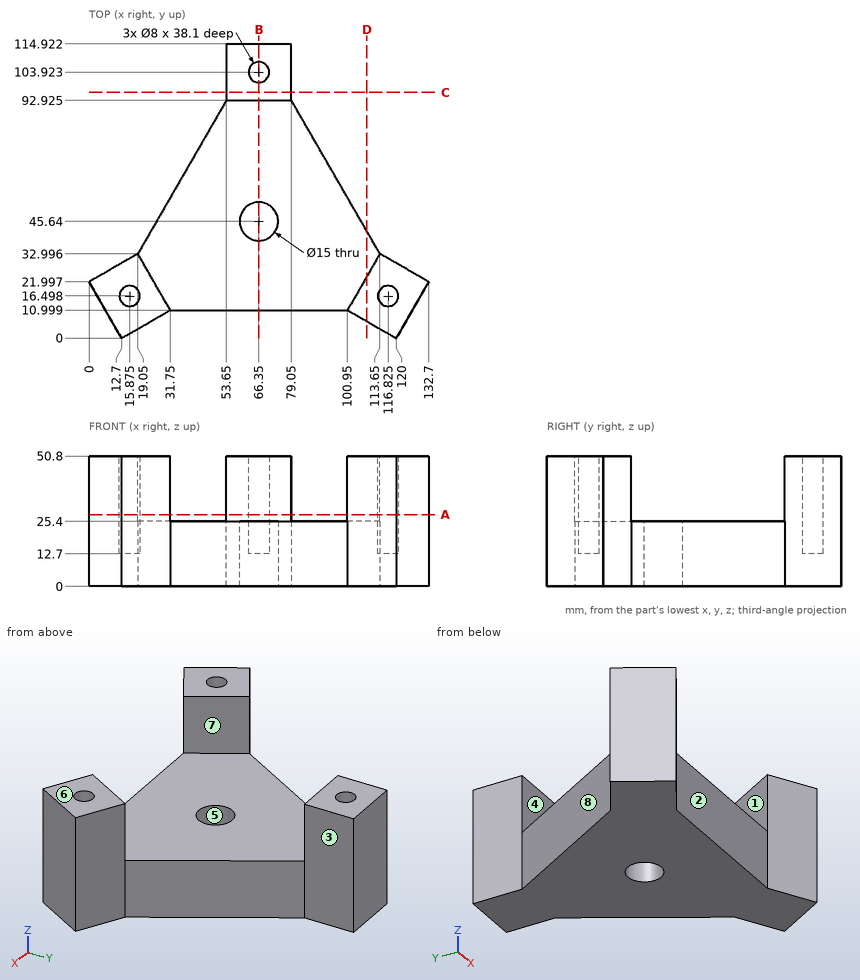
For this review, use the dimensioned drawing (mm, ordinates from the lowest corner) and the shaded views. A direction names the side the tool comes from. Give positions to 0.01 mm unless a question says otherwise; leave off trailing zeros. Order: outer loops, then holes, each group sorted by start corner. A loop starts at its lowest first (then second) coordinate and runs counter-clockwise, first axis right, second up. Notation, with made-up numbers: (7.5, -35) - (11.5, -35) arc R24 cw to (11.5, -18) - close; hole circle Ø5 at (-7, 73.5). An arc over 180 degrees is marked (long way). Use CSV: the item, a comma, the result in double quotes. Start each with the question number.
Q1. For P1, Ø1, axis at x = 46.5, y = 27.5, coming from the +Z side; P2, Ø1.5, axis at y = 94.5, z = 40, coming from the -X side; P3, Ø7, axis at x = 66.35, y = 103.92, coming from the +Z side, all flat-tipped, find the tip position at first contact; note any pin that passes through.
Q2. Machinability: for the marked faces 1, 2, 3 and 4, which of the approach directions +Z, -Z, +X, -X, +Y, -Y give a long, thin tool a straight path to every point of the face, cutting with its end or side? Answer none if there is none.
Q3. Take a section at A-A (z = 28). Count the separate pieces of the cut face and the enclosed holes in it, and give its area (3 significant figures).
Q4. For line 1 (Y direction, x = 66, z = 23); line 2 (Y direction, x = 66.35, z = 37) (1 decimal); line 3 (X direction, y = 104.5, z = 31.5), list the stretches that pass through material, from the lowest coordinate up.
Q5. Take a section at B-B (x = 66.35). State the section outline as (y, z) points (1 decimal), and give its area (3 significant figures).
Q6. Draft analysis for pull direction X (two halves, no side actions). For the marked faces 5, 6, 7 and 8, state which applies: pulls with the +X half, pulls with the -X half, needs draft (parallel to the pull), parting line crosses it, or undercut.
Q7. Take a section at D-D (x = 108.5). State the section outline as (y, z) points (1 decimal).
Q8. Take a section at C-C (y = 96). State the section outline as (x, z) points, and give its area (3 significant figures).
Calculated:
1,P1,"stops at z = 25.4"
1,P2,"stops at x = 53.65"
1,P3,"stops at z = 12.7"
2,face 1,"+Z, +Y"
2,face 2,"+Z, -Z, -Y"
2,face 3,"+Z, -Z, +X, +Y"
2,face 4,"+Z, +X, -X, -Y"
3,separate pieces,"3"
3,enclosed holes,"3"
3,area,"1,530 mm²"
4,line 1,"y = 11 to 38.15, 53.13 to 99.94, 107.91 to 114.92"
4,line 2,"y = 92.9 to 99.9, 107.9 to 114.9"
4,line 3,"x = 53.65 to 62.39, 70.31 to 79.05"
5,outline,"(11, 0) - (38.1, 0) - (38.1, 25.4) - (11, 25.4) - close; (53.1, 0) - (114.9, 0) - (114.9, 50.8) - (107.9, 50.8) - (107.9, 12.7) - (99.9, 12.7) - (99.9, 50.8) - (92.9, 50.8) - (92.9, 25.4) - (53.1, 25.4) - close"
5,area,"2,510 mm²"
6,face 5,"undercut"
6,face 6,"needs draft"
6,face 7,"undercut"
6,face 8,"pulls with the -X half"
7,outline,"(6.6, 0) - (41.9, 0) - (41.9, 25.4) - (24.1, 25.4) - (24.1, 50.8) - (6.6, 50.8) - close"
8,outline,"(53.65, 0) - (79.05, 0) - (79.05, 50.8) - (53.65, 50.8) - close"
8,area,"1,290 mm²"
